Build history of the part. All positions in model axes, mm. A direction names the side the tool comes from. Round coordinates to 2 decimals unless told otherwise and drop trailing zeros. Write each loop counter-clockwise with the first axis right and the second up, starting at its lowest first coordinate (ties: lowest second). Pieces come first, ordered by that corner, then holes. Notation, with made-up numbers: M -25,84.5 L -20,84.5 A15 cw -20,107.5 Z; hole C 83.25,-9.5 d3. An arc over 180 degrees is marked long. Use a Markdown table: item, result.
from build123d import *

# Parameters (mm, degrees)
F0_W         = 245
F0_H         = 200
F0_R         = 3.2
F0_W_2       = 215
F0_H_2       = 80
F1_DEPTH     = 3.175
F2_W         = 251.35
F2_H         = 206.35
F2_W_2       = 245
F2_H_2       = 200
F3_DEPTH     = 15
F4_SIZE      = 6.3
F6_R         = 3.3
F7_DEPTH     = 251.351
F8_R         = 3.3
F9_DEPTH     = 206.351
F10_T1_DEPTH = 263.75
F10_T3_DEPTH = 218.75


# Not quite as in the source:
# - a fillet or chamfer that OpenCascade refuses, or shapes differently, is made with other operations: its cross-section is extruded or revolved along the edge and cut away or added


with BuildPart() as f1:
    # F0 (on Top) → F1 (new body)
    with BuildSketch(Plane.XY):
        Rectangle(F0_W, F0_H)
        with Locations((-117.5, -70)):
            Circle(F0_R, mode=Mode.SUBTRACT)
        with Locations((117.5, -70)):
            Circle(F0_R, mode=Mode.SUBTRACT)
        with Locations((-117.5, 70)):
            Circle(F0_R, mode=Mode.SUBTRACT)
        Rectangle(F0_W_2, F0_H_2, mode=Mode.SUBTRACT)
        with Locations((117.5, 70)):
            Circle(F0_R, mode=Mode.SUBTRACT)
    extrude(amount=F1_DEPTH)

    # F2 (on face) → F3 (join)
    with BuildSketch(Plane(origin=(0, 0, 0), x_dir=(1, 0, 0), z_dir=(0, 0, -1))):
        Rectangle(F2_W, F2_H)
        Rectangle(F2_W_2, F2_H_2, mode=Mode.SUBTRACT)
    extrude(amount=-F3_DEPTH)

    # F4
    f4_edges = [f1.edges().sort_by_distance(p)[0] for p in [
        (-125.675, 103.175, 7.5),
        (125.675, 103.175, 7.5),
        (125.675, -103.175, 7.5),
        (-125.675, -103.175, 7.5),
    ]]
    chamfer(f4_edges, length=F4_SIZE)

    # F6 (on face) → F7 (cut, through all)
    with BuildSketch(Plane.YZ.offset(125.675)):
        with Locations((0, 10)):
            Circle(F6_R)
    extrude(amount=-F7_DEPTH, mode=Mode.SUBTRACT)

    # F8 (on face) → F9 (cut, through all)
    with BuildSketch(Plane(origin=(0, 103.175, 0), x_dir=(-1, 0, 0), z_dir=(0, 1, 0))):
        with Locations((0, 10)):
            Circle(F8_R)
    extrude(amount=-F9_DEPTH, mode=Mode.SUBTRACT)

    # F10: fillet of radius 5 on 4 edges, made by hand

    # F10_s2 → F10_t1 (cut)
    with BuildSketch(Plane.YZ.offset(-131.875)):
        with BuildLine():
            ThreePointArc((-98.175, 0), (-101.7105339059, 1.4644660941), (-103.175, 5))
            Line((-103.175, 5), (-103.175, 0))
            Line((-103.175, 0), (-98.175, 0))
        make_face()
        with BuildLine():
            ThreePointArc((98.175, 0), (101.7105339059, 1.4644660941), (103.175, 5))
            Line((103.175, 5), (103.175, 0))
            Line((103.175, 0), (98.175, 0))
        make_face()
    extrude(amount=F10_T1_DEPTH, mode=Mode.SUBTRACT)

    # F10_s4 → F10_t3 (cut)
    with BuildSketch(Plane.XZ.offset(-109.375)):
        with BuildLine():
            ThreePointArc((-120.675, 0), (-124.2105339059, 1.4644660941), (-125.675, 5))
            Line((-125.675, 5), (-125.675, 0))
            Line((-125.675, 0), (-120.675, 0))
        make_face()
        with BuildLine():
            ThreePointArc((120.675, 0), (124.2105339059, 1.4644660941), (125.675, 5))
            Line((125.675, 5), (125.675, 0))
            Line((125.675, 0), (120.675, 0))
        make_face()
    extrude(amount=F10_T3_DEPTH, mode=Mode.SUBTRACT)


solid = f1.part
Q1. Cut at D-D on x = 0. Give the cut face in (y, z) (3 decimals).
Response values:
| item | result |
|---|---|
| outline | M -103.175,5 A5 ccw -98.175,0 L -40,0 L -40,3.175 L -100,3.175 L -100,6.7 L -103.175,6.7 Z; M -103.175,13.3 L -100,13.3 L -100,15 L -103.175,15 Z; M 40,0 L 98.175,0 A5 ccw 103.175,5 L 103.175,6.7 L 100,6.7 L 100,3.175 L 40,3.175 Z; M 100,13.3 L 103.175,13.3 L 103.175,15 L 100,15 Z |
Q2. Drop flat-ended pins along their axis: P1, Ø1.6, axis at y = -19.5, z = 1.5, coming from the -X side; P2, Ø3.5, axis at y = 10.5, z = 2, coming from the +X side; P3, Ø5, axis at x = 117.5, y = 70, coming from the +Z side; P4, Ø1.6, axis at x = -48, z = 1.5, coming from the +Y side. Give the stop position or say it passes through.
Response values:
| item | result |
|---|---|
| P1 | stops at x = -124.88 |
| P2 | stops at x = 125.52 |
| P3 | passes through |
| P4 | stops at y = 102.38 |
Q3. Two-plate mould, pull along Y, no slides. Class faces 1 (the flat face through (-2, 46, 3.175)), 2 (the flat face through (-2, 103.175, 13)), 3 (the cylindrical face through (0.72, 101.61, 6.78)): +Y half, -Y half, draft (parallel to the pull), parting line (faces both ways), or undercut.
Response values:
| item | result |
|---|---|
| face 1 | undercut |
| face 2 | +Y half |
| face 3 | draft |
Q4. Cut at A-A on x = 38. Give the cut face in (y, z) (3 decimals).
Response values:
| item | result |
|---|---|
| outline | M -103.175,5 A5 ccw -98.175,0 L -40,0 L -40,3.175 L -100,3.175 L -100,15 L -103.175,15 Z; M 40,0 L 98.175,0 A5 ccw 103.175,5 L 103.175,15 L 100,15 L 100,3.175 L 40,3.175 Z |
Q5. Drill centre lines: L1, parallel to Y at x = 47, z = 5.25 (3 decimals); L2, parallel to X at y = 37.5, z = 4.5; L3, parallel to X at y = 85, z = 10.5 (3 decimals). Where is each one in solid material? Low to high.
Response values:
| item | result |
|---|---|
| L1 | y = -103.175 to -100, 100 to 103.175 |
| L2 | x = -125.65 to -122.5, 122.5 to 125.65 |
| L3 | x = -125.675 to -122.5, 122.5 to 125.675 |
Q6. Cut at C-C on y = 22. Give the cut face in (x, z) (3 decimals).
Response values:
| item | result |
|---|---|
| outline | M -125.675,5 A5 ccw -120.675,0 L -107.5,0 L -107.5,3.175 L -122.5,3.175 L -122.5,15 L -125.675,15 Z; M 107.5,0 L 120.675,0 A5 ccw 125.675,5 L 125.675,15 L 122.5,15 L 122.5,3.175 L 107.5,3.175 Z |
Q7. Cut at B-B on z = 10. Give the cut face in (x, y) (3 decimals), and give its area (3 significant figures).
Response values:
| item | result |
|---|---|
| outline | M -125.675,-96.875 L -119.375,-103.175 L -3.3,-103.175 L -3.3,-100 L -122.5,-100 L -122.5,-3.3 L -125.675,-3.3 Z; M -125.675,3.3 L -122.5,3.3 L -122.5,100 L -3.3,100 L -3.3,103.175 L -119.375,103.175 L -125.675,96.875 Z; M 3.3,-103.175 L 119.375,-103.175 L 125.675,-96.875 L 125.675,-3.3 L 122.5,-3.3 L 122.5,-100 L 3.3,-100 Z; M 3.3,100 L 122.5,100 L 122.5,3.3 L 125.675,3.3 L 125.675,96.875 L 119.375,103.175 L 3.3,103.175 Z |
| area | 2,700 mm2 |
Q8. Which spindle directions (+Z, -Z, +X, -X, +Y, -Y) get a long thin tool onto all of the face, cutting with end or side? Do faces 4 (the flat face through (123.27, 99.28, 7.57)), 5 (the flat face through (-2, -100, 6)). Say none if no direction does.
Response values:
| item | result |
|---|---|
| face 4 | +Z, -Z, +X, +Y |
| face 5 | +Z |
